CAD build for the part. Positions are in the model's coordinates, mm. A direction names the side the tool comes from. Give positions to 0.01 mm unless a question says otherwise; leave off trailing zeros. Write each loop counter-clockwise with the first axis right and the second up, starting at its lowest first coordinate (ties: lowest second). Pieces come first, ordered by that corner, then holes. Notation, with made-up numbers: (72.25, 66) - (101.25, 66) arc R23 cw to (101.25, 88) - close; hole circle Ø10 at (29, 6.25). An arc over 180 degrees is marked (long way). Put each result on its own line as item: value. Start each with the question number.
1. Drop flat-ended pins along their axis: pin 1 (3 mm diameter, centred on y = 1.5, z = -38, fed in from -X); pin 2 (2 mm diameter, centred on x = 55, y = 18.5, fed in from -Z); pin 3 (3 mm diameter, centred on x = 3.1, y = 5.5, fed in from +Z); pin 4 (8 mm diameter, centred on x = -11, y = 6.5, fed in from +Z). Give the stop position or say it passes through.
2. Cut at A-A on z = -75.5. List the corners of the cut face in (x, y), and give its area (3 significant figures).
3. Tool access for faces 1 (the cylindrical face through (1.479, 4.902, -48.866)), 2 (the flat face through (13, -6, -100.7)), 3 (the flat face through (13, 20.5, -95)), 4 (the flat face through (28, 0, -88)), 5 (the flat face through (2, 11, -90.87)): list every direction of +Z, -Z, +X, -X, +Y, -Y with a clear straight run to the whole face (end or side of a thin tool).
4. Wall check: line 1 (Y direction, x = 57.35, z = -23.75); line 2 (Y direction, x = 3.1, z = -83.25); line 3 (X direction, y = 2, z = -10.5). Give the ranges that are in metal, low to high.
5. Mould opens along X. For faces 6 (the cylindrical face through (51, 4, -79)), 7 (the flat face through (1, 16.5, -41)), 8 (the flat face through (58, 12, -27)) say: +X half, -X half, draft (parallel to the pull), parting line (faces both ways), or undercut.
6. Cut at B-B on x = 10.5. List the corners of the cut face in (y, z), and give its area (3 significant figures).
from build123d import *

# Parameters (mm, degrees)
AUFSATZ_LINEAR_AUSTRAGEN1_DEPTH      = 20.5
SCHNITT_LINEAR_AUSTRAGEN1_DEPTH      = 85.1
SKIZZE3_R                            = 3.1
SCHNITT_LINEAR_AUSTRAGEN2_DEPTH      = 87.42
SCHNITT_LINEAR_AUSTRAGEN3_DEPTH      = 2
SKIZZE5_R                            = 0.75
SCHNITT_LINEAR_AUSTRAGEN4_DEPTH      = 2
AUFSATZ_LINEAR_AUSTRAGEN2_DEPTH      = 20.5
SKIZZE7_W                            = 9.5
SKIZZE7_H                            = 20.5
AUFSATZ_LINEAR_AUSTRAGEN3_DEPTH      = 25.87
SCHNITT_LINEAR_AUSTRAGEN5_DEPTH      = 18.09
SKIZZE9_R                            = 1.75
SCHNITT_LINEAR_AUSTRAGEN6_DEPTH      = 24.9
AUFSATZ_LINEAR_AUSTRAGEN4_DEPTH      = 60
AUFSATZ_LINEAR_AUSTRAGEN5_DEPTH      = 40
AUFSATZ_LINEAR_AUSTRAGEN5_DEPTH_BACK = 70
AUFSATZ_LINEAR_AUSTRAGEN6_DEPTH      = 4
AUFSATZ_LINEAR_AUSTRAGEN7_DEPTH      = 4
AUFSATZ_LINEAR_AUSTRAGEN8_DEPTH      = 28.4
SCHNITT_LINEAR_AUSTRAGEN7_DEPTH      = 3


with BuildPart() as part:
    # Skizze1 → Aufsatz-Linear austragen1 (new body)
    with BuildSketch(Plane(origin=(0, 0, 0), x_dir=(1, 0, 0), z_dir=(0, 1, 0))):
        with BuildLine():
            Line((0, 54.3), (0, 0))
            Line((0, 0), (3, 0))
            Line((3, 0), (3, 51.3))
            ThreePointArc((3, 51.3), (4.376598128, 54.623401872), (7.7, 56))
            Line((7.7, 56), (50.3, 56))
            ThreePointArc((50.3, 56), (53.623401872, 54.623401872), (55, 51.3))
            Line((55, 51.3), (55, 0))
            Line((55, 0), (58, 0))
            Line((58, 0), (58, 54.3))
            ThreePointArc((58, 54.3), (56.623401872, 57.623401872), (53.3, 59))
            Line((53.3, 59), (4.7, 59))
            ThreePointArc((4.7, 59), (1.376598128, 57.623401872), (0, 54.3))
        make_face()
    extrude(amount=AUFSATZ_LINEAR_AUSTRAGEN1_DEPTH)

    # Skizze2 → Schnitt-Linear austragen1 (cut)
    with BuildSketch(Plane(origin=(58, 0, 0), x_dir=(0, 0, -1), z_dir=(1, 0, 0))):
        with BuildLine():
            ThreePointArc((0, 10.25), (3.002155493, 17.497844507), (10.25, 20.5))
            Line((10.25, 20.5), (0, 20.5))
            Line((0, 20.5), (0, 10.25))
        make_face()
        with BuildLine():
            ThreePointArc((10.25, 0), (3.002155493, 3.002155493), (0, 10.25))
            Line((0, 10.25), (0, 0))
            Line((0, 0), (10.25, 0))
        make_face()
    extrude(amount=-SCHNITT_LINEAR_AUSTRAGEN1_DEPTH, mode=Mode.SUBTRACT)

    # Skizze3 → Schnitt-Linear austragen2 (cut)
    with BuildSketch(Plane(origin=(58, 0, 0), x_dir=(0, 0, -1), z_dir=(1, 0, 0))):
        with Locations((10.25, 10.25)):
            Circle(SKIZZE3_R)
    extrude(amount=-SCHNITT_LINEAR_AUSTRAGEN2_DEPTH, mode=Mode.SUBTRACT)

    # Skizze4 → Schnitt-Linear austragen3 (cut)
    with BuildSketch(Plane.ZY.offset(-55)):
        with BuildLine():
            Line((-12.895262454, 4.367384373), (-27.5, 7.5))
            ThreePointArc((-27.5, 7.5), (-30, 10), (-27.5, 12.5))
            Line((-27.5, 12.5), (-13.215100612, 15.978067599))
            ThreePointArc((-13.215100612, 15.978067599), (-3.802439634, 10.427610206), (-12.895262454, 4.367384373))
        make_face()
    extrude(amount=-SCHNITT_LINEAR_AUSTRAGEN3_DEPTH, mode=Mode.SUBTRACT)

    # Skizze5 → Schnitt-Linear austragen4 (cut)
    with BuildSketch(Plane.ZY.offset(-57)):
        with Locations((-26.749999999, 10.249909889)):
            Circle(SKIZZE5_R)
        with Locations((-23.75, 10.25)):
            Circle(SKIZZE5_R)
        with Locations((-20.75, 10.25)):
            Circle(SKIZZE5_R)
        with Locations((-17.75, 10.25)):
            Circle(SKIZZE5_R)
    extrude(amount=-SCHNITT_LINEAR_AUSTRAGEN4_DEPTH, mode=Mode.SUBTRACT)

    # Skizze6 → Aufsatz-Linear austragen2 (add, through all)
    with BuildSketch(Plane.XZ):
        with BuildLine():
            Line((29, -59), (2.2, -59))
            ThreePointArc((2.2, -59), (-1.123401872, -60.376598128), (-2.5, -63.7))
            Line((-2.5, -63.7), (-2.5, -65))
            Line((-2.5, -65), (27.5, -65))
            Line((27.5, -65), (57.5, -65))
            Line((57.5, -65), (57.5, -63.7))
            ThreePointArc((57.5, -63.7), (56.123401872, -60.376598128), (52.8, -59))
            Line((52.8, -59), (29, -59))
        make_face()
    extrude(amount=-AUFSATZ_LINEAR_AUSTRAGEN2_DEPTH)

    # Skizze7 → Aufsatz-Linear austragen3 (add)
    with BuildSketch(Plane(origin=(0, 0, -65), x_dir=(-1, 0, 0), z_dir=(0, 0, -1))):
        with Locations((-52.75, 10.25)):
            Rectangle(SKIZZE7_W, SKIZZE7_H)
        with Locations((-2.25, 10.25)):
            Rectangle(SKIZZE7_W, SKIZZE7_H)
    extrude(amount=AUFSATZ_LINEAR_AUSTRAGEN3_DEPTH)

    # Skizze8 → Schnitt-Linear austragen5 (cut)
    with BuildSketch(Plane.ZY.offset(2.5)):
        with BuildLine():
            Line((-83.87, 14.5), (-67.2, 14.5))
            ThreePointArc((-67.2, 14.5), (-65.785786438, 13.914213562), (-65.2, 12.5))
            Line((-65.2, 12.5), (-65.2, 8))
            ThreePointArc((-65.2, 8), (-65.785786438, 6.585786438), (-67.2, 6))
            Line((-67.2, 6), (-83.87, 6))
            ThreePointArc((-83.87, 6), (-85.284213562, 6.585786438), (-85.87, 8))
            Line((-85.87, 8), (-85.87, 12.5))
            ThreePointArc((-85.87, 12.5), (-85.284213562, 13.914213562), (-83.87, 14.5))
        make_face()
    extrude(amount=-SCHNITT_LINEAR_AUSTRAGEN5_DEPTH, mode=Mode.SUBTRACT)

    # Skizze9 → Schnitt-Linear austragen6 (cut)
    with BuildSketch(Plane(origin=(0, 0, -90.87), x_dir=(-1, 0, 0), z_dir=(0, 0, -1))):
        with Locations((-3.1, 5.5)):
            Circle(SKIZZE9_R)
        with Locations((-3.1, 15.5)):
            Circle(SKIZZE9_R)
        with Locations((-51.9, 5.5)):
            Circle(SKIZZE9_R)
        with Locations((-51.9, 15.5)):
            Circle(SKIZZE9_R)
    extrude(amount=-SCHNITT_LINEAR_AUSTRAGEN6_DEPTH, mode=Mode.SUBTRACT)

    # Skizze10 → Aufsatz-Linear austragen4 (add, through all)
    with BuildSketch(Plane(origin=(57.5, 0, 0), x_dir=(0, 0, -1), z_dir=(1, 0, 0))):
        with BuildLine():
            Line((90.87, 20.5), (84.87, 20.5))
            Line((84.87, 20.5), (84.87, 22.5))
            ThreePointArc((84.87, 22.5), (85.455786438, 23.914213562), (86.87, 24.5))
            Line((86.87, 24.5), (90.87, 24.5))
            Line((90.87, 24.5), (90.87, 20.5))
        make_face()
        with BuildLine():
            Line((90.87, 0), (84.87, 0))
            Line((84.87, 0), (84.87, -2))
            ThreePointArc((84.87, -2), (85.455786438, -3.414213562), (86.87, -4))
            Line((86.87, -4), (90.87, -4))
            Line((90.87, -4), (90.87, 0))
        make_face()
    extrude(amount=-AUFSATZ_LINEAR_AUSTRAGEN4_DEPTH)

    # Skizze11 → Aufsatz-Linear austragen5 (add, two sides: drawn at the far end of the back side and taken through both)
    with BuildSketch(Plane.ZY.offset(2.5).offset(-AUFSATZ_LINEAR_AUSTRAGEN5_DEPTH_BACK)):
        with BuildLine():
            Line((-90.87, 24.5), (-100.7, 24.5))
            Line((-100.7, 24.5), (-100.7, 28.6))
            ThreePointArc((-100.7, 28.6), (-100.963603897, 29.236396103), (-101.6, 29.5))
            Line((-101.6, 29.5), (-101.8, 29.5))
            ThreePointArc((-101.8, 29.5), (-102.436396103, 29.236396103), (-102.7, 28.6))
            Line((-102.7, 28.6), (-102.7, 22.4))
            ThreePointArc((-102.7, 22.4), (-102.143502884, 21.056497116), (-100.8, 20.5))
            Line((-100.8, 20.5), (-100.7, 20.5))
            Line((-100.7, 20.5), (-90.87, 20.5))
            Line((-90.87, 20.5), (-90.87, 24.5))
        make_face()
        with BuildLine():
            Line((-90.87, -4), (-100.7, -4))
            Line((-100.7, -4), (-100.7, -7.8))
            ThreePointArc((-100.7, -7.8), (-100.963603897, -8.436396103), (-101.6, -8.7))
            Line((-101.6, -8.7), (-101.8, -8.7))
            ThreePointArc((-101.8, -8.7), (-102.436396103, -8.436396103), (-102.7, -7.8))
            Line((-102.7, -7.8), (-102.7, -1.6))
            ThreePointArc((-102.7, -1.6), (-102.143502884, -0.256497116), (-100.8, 0.3))
            Line((-100.8, 0.3), (-100.7, 0.3))
            Line((-100.7, 0.3), (-90.87, 0.3))
            Line((-90.87, 0.3), (-90.87, -4))
        make_face()
    extrude(amount=AUFSATZ_LINEAR_AUSTRAGEN5_DEPTH + AUFSATZ_LINEAR_AUSTRAGEN5_DEPTH_BACK)

    # Skizze12 → Aufsatz-Linear austragen6 (add)
    with BuildSketch(Plane(origin=(0, 24.5, 0), x_dir=(1, 0, 0), z_dir=(0, 1, 0))):
        with BuildLine():
            Line((-42.5, 90.87), (-2.5, 90.87))
            Line((-2.5, 90.87), (-2.5, 86.87))
            add(Edge.make_bspline(
                [(-42.5, 90.87), (-9.080607123, 90.092835271), (-2.5, 86.87)],
                knots=[0, 0, 0, 1, 1, 1], degree=2))
        make_face()
    extrude(amount=-AUFSATZ_LINEAR_AUSTRAGEN6_DEPTH)

    # Skizze13 → Aufsatz-Linear austragen7 (add)
    with BuildSketch(Plane.XZ.offset(4)):
        with BuildLine():
            Line((-2.5, -86.87), (-2.5, -90.87))
            Line((-2.5, -90.87), (-42.5, -90.87))
            add(Edge.make_bspline(
                [(-42.5, -90.87), (-8.320155044, -89.830707386), (-2.5, -86.87)],
                knots=[0, 0, 0, 1, 1, 1], degree=2))
        make_face()
    extrude(amount=-AUFSATZ_LINEAR_AUSTRAGEN7_DEPTH)

    # Skizze14 → Aufsatz-Linear austragen8 (add)
    with BuildSketch(Plane.XZ.offset(4)):
        with BuildLine():
            Line((57.5, -86.87), (57.5, -90.87))
            Line((57.5, -90.87), (67.5, -90.87))
            add(Edge.make_bspline(
                [(57.5, -86.87), (60.425368179, -89.995001665), (67.5, -90.87)],
                knots=[0, 0, 0, 1, 1, 1], degree=2))
        make_face()
    extrude(amount=-AUFSATZ_LINEAR_AUSTRAGEN8_DEPTH)

    # Skizze16 → Schnitt-Linear austragen7 (cut)
    with BuildSketch(Plane.ZY):
        with BuildLine():
            Line((-46.721244461, 4), (-35.100330168, 4))
            ThreePointArc((-35.100330168, 4), (-32.979009824, 4.878679656), (-32.100330168, 7))
            Line((-32.100330168, 7), (-32.100330168, 13.5))
            ThreePointArc((-32.100330168, 13.5), (-32.979009824, 15.621320344), (-35.100330168, 16.5))
            Line((-35.100330168, 16.5), (-46.721244461, 16.5))
            ThreePointArc((-46.721244461, 16.5), (-48.842564804, 15.621320344), (-49.721244461, 13.5))
            Line((-49.721244461, 13.5), (-49.721244461, 7))
            ThreePointArc((-49.721244461, 7), (-48.842564804, 4.878679656), (-46.721244461, 4))
        make_face()
    extrude(amount=-SCHNITT_LINEAR_AUSTRAGEN7_DEPTH, mode=Mode.SUBTRACT)


solid = part.part
Report:
1. pin 1: stops at x = 0
1. pin 2: stops at z = -90.87
1. pin 3: stops at z = -0.53
1. pin 4: passes through
2. outline: (-2.5, 0) - (7, 0) - (7, 6) - (4.78, 6) arc R1.75 cw (long way) to (1.42, 6) - (-2.5, 6) - close; (-2.5, 14.5) - (1.66, 14.5) arc R1.75 cw (long way) to (4.54, 14.5) - (7, 14.5) - (7, 20.5) - (-2.5, 20.5) - close; (48, 0) - (57.5, 0) - (57.5, 20.5) - (48, 20.5) - close; hole circle Ø3.5 at (51.9, 5.5); hole circle Ø3.5 at (51.9, 15.5)
2. area: 275 mm²
3. face 1: -X
3. face 2: +Z, +X, -X, -Y
3. face 3: -Z
3. face 4: none
3. face 5: -Z, +X, -X
4. line 1: y = 0 to 9.5, 11 to 20.5
4. line 2: y = 0 to 3.75, 17.25 to 20.5
4. line 3: x = 0 to 3, 55 to 58
5. face 6: undercut
5. face 7: draft
5. face 8: +X half
6. outline: (-8.7, -101.8) arc R0.9 ccw to (-7.8, -102.7) - (-1.6, -102.7) arc R1.9 ccw to (0.3, -100.8) - (0.3, -90.87) - (0, -90.87) - (0, -84.87) - (-2, -84.87) arc R2 ccw to (-4, -86.87) - (-4, -100.7) - (-7.8, -100.7) arc R0.9 ccw to (-8.7, -101.6) - close; (0, -65) - (20.5, -65) - (20.5, -56) - (0, -56) - close; (20.5, -100.8) arc R1.9 ccw to (22.4, -102.7) - (28.6, -102.7) arc R0.9 ccw to (29.5, -101.8) - (29.5, -101.6) arc R0.9 ccw to (28.6, -100.7) - (24.5, -100.7) - (24.5, -86.87) arc R2 ccw to (22.5, -84.87) - (20.5, -84.87) - close
6. area: 346 mm²
